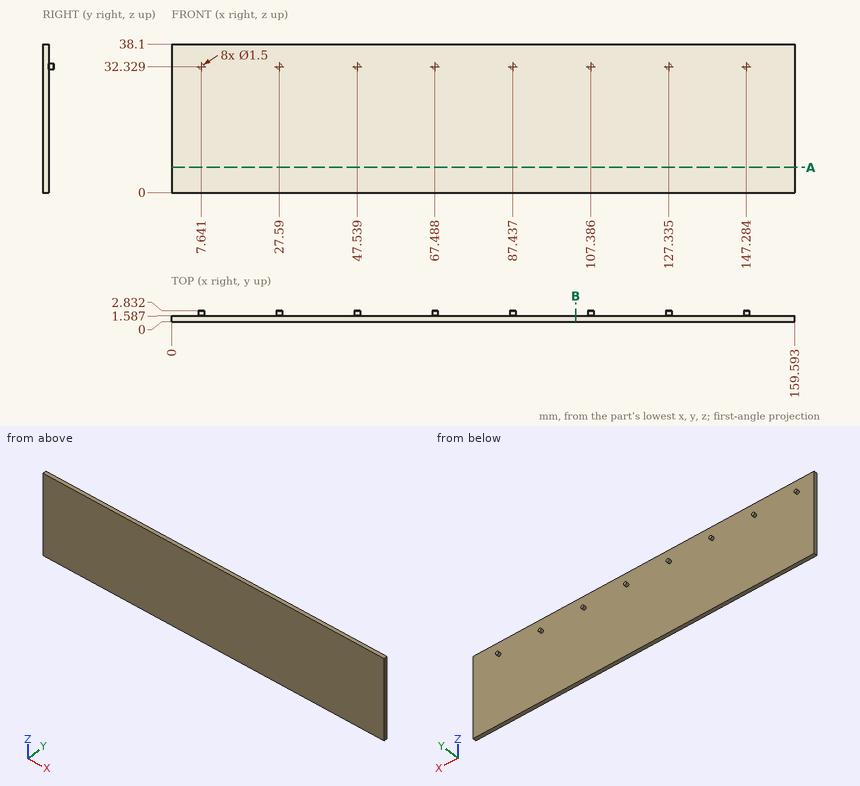
Print and shaded views of the part. All mm, measured from the part's lowest x, y and z. Give positions to 0.01 mm unless a question says otherwise; leave off trailing zeros. Loops run counter-clockwise (first coordinate to the right, second up) from the corner with the lowest first, then second, coordinate; pieces in that order, holes last. Notation, with made-up numbers: M 75,-11 L 110,-11 A19 ccw 110,2 Z; hole C 55.25,-3 d10. An arc over 180 degrees is marked long. Write each question's results on one line, items separated by ' | '.
Q1. Flat gauge pin, fed straight in: P1, Ø3, axis at x = 72, z = 14.5, coming from the +Y side. Where does the tip first touch, or does it go through?
Geometry check:
P1: stops at y = 1.59
Q2. Probe probe 1 along Y at (x, z) = (129, 11.5); probe 2 along Z at (x, y) = (107, 2.3) (1 decimal). List the from-to ranges inside material, lowest first.
Geometry check:
probe 1: y = 0 to 1.59 | probe 2: z = 31.7 to 33
Q3. Band-saw the part on B-B on x = 103.5. Write the cut outline in (y, z).
Geometry check:
outline: M 0,0 L 1.59,0 L 1.59,38.1 L 0,38.1 Z
Q4. Band-saw the part on A-A on z = 6.5. Write the cut outline in (x, y).
Geometry check:
outline: M 0,0 L 159.59,0 L 159.59,1.59 L 0,1.59 Z
